Read the model definition and answer for the solid it produces. Units are mm, in the model's axes. A direction names the side the tool comes from. Round coordinates to 2 decimals unless told otherwise and drop trailing zeros. Loops run counter-clockwise (first coordinate to the right, second up) from the corner with the lowest first, then second, coordinate; pieces in that order, holes last. Notation, with made-up numbers: M 49.5,-1 L 58.5,-1 A27 cw 58.5,35 Z; hole C 64,-35.5 d8. An arc over 180 degrees is marked long. Write each question's results on one line, items separated by ' | '.
```python
from build123d import *

# Parameters (mm, degrees)
SKETCH1_W                      = 96
SKETCH1_H                      = 96
BOSS_EXTRUDE1_DEPTH            = 8
SKETCH2_W                      = 92
SKETCH2_H                      = 92
COMPONENT_PLATFORM_DEPTH       = 6
CABLE_SLOTS_DEPTH              = 6
INNER_CORNER_FILLETS_R         = 3
M3X0_5_TAPPED_HOLE1_AT_2_COUNT = 2
M3X0_5_TAPPED_HOLE1_AT_2_PITCH = 70
M3X0_5_TAPPED_HOLE2_AT_2_COUNT = 2
M3X0_5_TAPPED_HOLE2_AT_2_PITCH = 70
F_1_0MM_DOWEL_HOLE1_D          = 1
F_1_0MM_DOWEL_HOLE1_DEPTH      = 3.7
F_1_0MM_DOWEL_HOLE1_TIP        = 0.30043031
SKETCH29_R                     = 12
HDD_EXTRUSION_CUTOUT_DEPTH     = 10
HDD_EXTRUSION_CUTOUT_2_DEPTH   = 10
F_3_0MM_DOWEL_HOLE1_D          = 3
F_3_0MM_DOWEL_HOLE1_DEPTH      = 2
F_3_0MM_DOWEL_HOLE2_D          = 3


with BuildPart() as part:
    # Sketch1 → Boss-Extrude1 (new body)
    with BuildSketch(Plane.XY):
        Rectangle(SKETCH1_W, SKETCH1_H)
    extrude(amount=BOSS_EXTRUDE1_DEPTH)

    # Sketch2 → Component Platform (cut)
    with BuildSketch(Plane.XY.offset(8)):
        Rectangle(SKETCH2_W, SKETCH2_H)
    extrude(amount=-COMPONENT_PLATFORM_DEPTH, mode=Mode.SUBTRACT)

    # Sketch3 → Cable Slots (cut, symmetric)
    with BuildSketch(Plane.XY.offset(2)):
        with BuildLine():
            Line((-33.878679656, -25.121320344), (-28.878679656, -20.121320344))
            ThreePointArc((-28.878679656, -20.121320344), (-28.228361402, -19.148050297), (-28, -18))
            Line((-28, -18), (-28, 18))
            ThreePointArc((-28, 18), (-28.228361402, 19.148050297), (-28.878679656, 20.121320344))
            Line((-28.878679656, 20.121320344), (-33.878679656, 25.121320344))
            ThreePointArc((-33.878679656, 25.121320344), (-34.851949703, 25.771638598), (-36, 26))
            Line((-36, 26), (-48, 26))
            Line((-48, 26), (-48, -26))
            Line((-48, -26), (-36, -26))
            ThreePointArc((-36, -26), (-34.851949703, -25.771638598), (-33.878679656, -25.121320344))
        make_face()
        with BuildLine():
            Line((48, -26), (48, 26))
            Line((48, 26), (36, 26))
            ThreePointArc((36, 26), (34.851949703, 25.771638598), (33.878679656, 25.121320344))
            Line((33.878679656, 25.121320344), (28.878679656, 20.121320344))
            ThreePointArc((28.878679656, 20.121320344), (28.228361402, 19.148050297), (28, 18))
            Line((28, 18), (28, -18))
            ThreePointArc((28, -18), (28.228361402, -19.148050297), (28.878679656, -20.121320344))
            Line((28.878679656, -20.121320344), (33.878679656, -25.121320344))
            ThreePointArc((33.878679656, -25.121320344), (34.851949703, -25.771638598), (36, -26))
            Line((36, -26), (48, -26))
        make_face()
    extrude(amount=CABLE_SLOTS_DEPTH, both=True, mode=Mode.SUBTRACT)

    # Inner Corner Fillets
    inner_corner_fillets_edges = [part.edges().sort_by_distance(p)[0] for p in [
        (-46, -46, 5),
        (-46, 46, 5),
        (46, 46, 5),
        (46, -46, 5),
    ]]
    fillet(inner_corner_fillets_edges, radius=INNER_CORNER_FILLETS_R)

    # Sketch14 → M3x0.5 Tapped Hole1 (revolve, cut)
    with BuildSketch(Plane(origin=(48, -35, 5), x_dir=(0, 0, -1), z_dir=(0, 1, 0))):
        Polygon((0, 0), (0, 10.751075774), (1.25, 10), (1.25, 0), align=None)
    m3x0_5_tapped_hole1 = revolve(axis=Axis((54.35, -35, 5), (-1, 0, 0)), mode=Mode.SUBTRACT)

    # M3x0.5 Tapped Hole1 at 2: M3x0.5 Tapped Hole1 ×2
    with Locations(*[(0, i * M3X0_5_TAPPED_HOLE1_AT_2_PITCH, 0) for i in range(1, M3X0_5_TAPPED_HOLE1_AT_2_COUNT)]):
        add(m3x0_5_tapped_hole1, mode=Mode.SUBTRACT)

    # Sketch16 → M3x0.5 Tapped Hole2 (revolve, cut)
    with BuildSketch(Plane(origin=(35, 48, 5), x_dir=(0, 0, 1), z_dir=(1, 0, 0))):
        Polygon((0, 0), (0, 10.751075774), (1.25, 10), (1.25, 0), align=None)
    m3x0_5_tapped_hole2 = revolve(axis=Axis((35, 54.35, 5), (0, -1, 0)), mode=Mode.SUBTRACT)

    # M3x0.5 Tapped Hole2 at 2: M3x0.5 Tapped Hole2 ×2
    with Locations(*[(-i * M3X0_5_TAPPED_HOLE2_AT_2_PITCH, 0, 0) for i in range(1, M3X0_5_TAPPED_HOLE2_AT_2_COUNT)]):
        add(m3x0_5_tapped_hole2, mode=Mode.SUBTRACT)

    # Mirror1: M3x0.5 Tapped Hole1 across plane
    add(m3x0_5_tapped_hole1.mirror(Plane(origin=(0, 0, 0), x_dir=(0, 0, 1), z_dir=(1, 0, 0))), mode=Mode.SUBTRACT)

    # Mirror1 copy 1 sketch → Mirror1 copy 1 (revolve, cut)
    with BuildSketch(Plane(origin=(-48, 35, 5), x_dir=(0, 0, -1), z_dir=(0, 1, 0))):
        Polygon((0, 0), (0, -10.751075774), (1.25, -10), (1.25, 0), align=None)
    revolve(axis=Axis((-54.35, 35, 5), (-1, 0, 0)), mode=Mode.SUBTRACT)

    # Mirror2: M3x0.5 Tapped Hole2 across plane
    add(m3x0_5_tapped_hole2.mirror(Plane(origin=(0, 0, 0), x_dir=(0, 0, 1), z_dir=(0, -1, 0))), mode=Mode.SUBTRACT)

    # Mirror2 copy 1 sketch → Mirror2 copy 1 (revolve, cut)
    with BuildSketch(Plane(origin=(-35, -48, 5), x_dir=(0, 0, 1), z_dir=(1, 0, 0))):
        Polygon((0, 0), (0, -10.751075774), (1.25, -10), (1.25, 0), align=None)
    revolve(axis=Axis((-35, -54.35, 5), (0, -1, 0)), mode=Mode.SUBTRACT)

    # Ø1.0mm Dowel Hole1
    with Locations(Plane.XY.offset(2)):
        with Locations((-19.31998517, -29.75), (24.78001483, -32.85), (-22.91998517, 32.85)):
            Hole(F_1_0MM_DOWEL_HOLE1_D / 2, depth=F_1_0MM_DOWEL_HOLE1_DEPTH)
            with Locations((0, 0, -(F_1_0MM_DOWEL_HOLE1_DEPTH + F_1_0MM_DOWEL_HOLE1_TIP / 2))):  # 118° drill point
                Cone(0, F_1_0MM_DOWEL_HOLE1_D / 2, F_1_0MM_DOWEL_HOLE1_TIP, mode=Mode.SUBTRACT)

    # Sketch29 → HDD Extrusion Cutout (cut)
    with BuildSketch(Plane(origin=(0, 0, 0), x_dir=(-1, 0, 0), z_dir=(0, 0, -1))):
        with Locations((-0.08192631, -8.74785827)):
            Circle(SKETCH29_R)
    extrude(amount=-HDD_EXTRUSION_CUTOUT_DEPTH, mode=Mode.SUBTRACT)

    # Sketch9 → HDD Extrusion Cutout 2 (cut)
    with BuildSketch(Plane.XY.offset(2)):
        with BuildLine():
            Line((25, 31), (25, 15))
            ThreePointArc((25, 15), (24.414213562, 13.585786438), (23, 13))
            Line((23, 13), (7, 13))
            ThreePointArc((7, 13), (5.585786438, 13.585786438), (5, 15))
            Line((5, 15), (5, 31))
            ThreePointArc((5, 31), (5.585786438, 32.414213562), (7, 33))
            Line((7, 33), (23, 33))
            ThreePointArc((23, 33), (24.414213562, 32.414213562), (25, 31))
        make_face()
    extrude(amount=-HDD_EXTRUSION_CUTOUT_2_DEPTH, mode=Mode.SUBTRACT)

    # Ø3.0mm Dowel Hole1
    with Locations(Plane.XY.offset(2)):
        with Locations((-31.790998517, -39.06), (31.29001483, -39.06), (31.29001483, 38.94), (-31.790998517, 38.94)):
            Hole(F_3_0MM_DOWEL_HOLE1_D / 2, depth=F_3_0MM_DOWEL_HOLE1_DEPTH)

    # Ø3.0mm Dowel Hole2 (through all)
    with Locations(Plane.XY.offset(2)):
        with Locations((40, -40), (-40, -40), (-40, 40), (40, 40)):
            Hole(F_3_0MM_DOWEL_HOLE2_D / 2)


solid = part.part
```
1. Find the intervals of material crossed by L1, parallel to X at y = 41, z = 6.25; L2, parallel to Y at x = -40, z = 1.05, in increasing order.
Completed:
L1: x = -48 to -46, 46 to 48 | L2: y = -48 to -41.5, -38.5 to -26, 26 to 38.5, 41.5 to 48
2. Given P1, Ø3, axis at y = 35, z = 5, coming from the +X side; P2, Ø1, axis at x = 29.5, y = 4, coming from the +Z side; P3, Ø1.6, axis at y = 22, z = 1, coming from the -X side; P4, Ø3.5, axis at x = 31.29, y = 38.94, coming from the +Z side, each flat-ended and moving along its own axis, determine where each tip first touches the part or whether it passes through.
Completed:
P1: stops at x = 48 | P2: passes through | P3: stops at x = -31.56 | P4: stops at z = 2
3. Find section B-B, the plane x = -40. Give the vertices of the cut face in (y, z).
Completed:
outline: M -48,0 L -41.5,0 L -41.5,2 L -46,2 L -46,8 L -48,8 Z; M -38.5,0 L -26,0 L -26,2 L -38.5,2 Z; M 26,0 L 38.5,0 L 38.5,2 L 26,2 Z; M 41.5,0 L 48,0 L 48,8 L 46,8 L 46,2 L 41.5,2 Z
4. Determine the mould class of faces 5 (the face through (-47.01, 33.76, 5.16)), 6 (the face through (-33.78, -47.01, 4.73)), 7 (the face through (-1, 48, 4)) for opening direction Y: released by +Y, released by -Y, zero draft, split by the parting line, or undercut.
Completed:
face 5: undercut | face 6: zero draft | face 7: released by +Y
5. Which of the six approach directions +Z, -Z, +X, -X, +Y, -Y give full straight-line access (tool end or side, diameter ignored) to faces 1 (the face through (46, -34.6, 6.4)), 2 (the face through (31.414, 22.656, 1.014)), 3 (the face through (-48, -37, 4)), 4 (the face through (-43.7, 26, 1.6))?
Completed:
face 1: +Z | face 2: +Z, -Z, +X | face 3: +Z, -Z, -X, +Y, -Y | face 4: +Z, -Z, -X
6. Find section A-A, the plane y = 28. Give the vertices of the cut face in (x, z), then the cut area to 3 significant figures.
Completed:
outline: M -48,0 L 5,0 L 5,2 L -46,2 L -46,8 L -48,8 Z; M 25,0 L 48,0 L 48,8 L 46,8 L 46,2 L 25,2 Z | area: 176 mm2
